Here's how the part is built. I have some questions about the finished solid (model axes, mm). A direction names the side the tool comes from. Give positions to 0.01 mm unless a question says otherwise; leave off trailing zeros. Order: outer loops, then holes, each group sorted by start corner. A loop starts at its lowest first (then second) coordinate and runs counter-clockwise, first axis right, second up. Notation, with made-up numbers: (8, 78.25) - (41, 78.25) arc R34 ccw to (41, 116.25) - close; hole circle Ø2 at (-27, -6.75). An arc over 180 degrees is marked (long way). One line per question, with ' | ' between items.
from build123d import *

# Parameters (mm, degrees)
SKETCH1_R           = 2
BOSS_EXTRUDE1_DEPTH = 3.3
SKETCH2_R           = 2
CUT_EXTRUDE1_DEPTH  = 513.420535354
SKETCH3_R           = 2
CUT_EXTRUDE2_DEPTH  = 4


with BuildPart() as part:
    # Sketch1 → Boss-Extrude1 (new body)
    with BuildSketch(Plane.XY):
        Polygon((327.436217585, 0.003466677), (121.498383462, 0.003466677), (108.169003487, 28.58841428), (-63.446663307, -51.437285405), (-52.881206764, -74.094980081), (-74.632593653, -84.237818363), (36.177914576, -321.871720124), (57.929301464, -311.728881842), (398.70102939, -152.824415428), align=None)
        with Locations(Location((372.759364157, -134.57831982, 0), (0, 0, 180))):
            Circle(SKETCH1_R, mode=Mode.SUBTRACT)
    extrude(amount=BOSS_EXTRUDE1_DEPTH)

    # Sketch2 → Cut-Extrude1 (cut, through all)
    with BuildSketch(Plane.XY.offset(3.3)):
        with Locations((105.144723808, 16.144390316)):
            Circle(SKETCH2_R)
        with Locations((-26.593400357, -45.286105853)):
            Circle(SKETCH2_R)
    extrude(amount=-CUT_EXTRUDE1_DEPTH, mode=Mode.SUBTRACT)

    # Sketch3 → Cut-Extrude2 (cut)
    with BuildSketch(Plane.XY.offset(3.3)):
        with Locations((45.851705082, -295.293199148)):
            Circle(SKETCH3_R)
        with Locations((63.977860822, -286.840833914)):
            Circle(SKETCH3_R)
    extrude(amount=-CUT_EXTRUDE2_DEPTH, mode=Mode.SUBTRACT)


solid = part.part
1) I'm going to push flat-ended pins straight in: P1, Ø1, axis at x = -18.5, y = -41, coming from the -Z side; P2, Ø3.5, axis at x = 63.98, y = -286.84, coming from the +Z side; P3, Ø1.5, axis at x = 280.5, z = 3, coming from the +Y side; P4, Ø1, axis at y = -181.5, z = 1, coming from the +X side. Where does each tip first touch, or does it pass through?
Model answer:
P1: stops at z = 0 | P2: passes through | P3: stops at y = 0 | P4: stops at x = 338.28
2) On a 3-axis mill with a long thin cutter (end or side, diameter ignored), from which of +Z, -Z, +X, -X, +Y, -Y can I reach the whole of each face in a straight line? I mean faces 1 (the face through (-20, -201.4, 1.6)), 2 (the face through (-63.605, -79.095, 1.627)). Say none if no direction works.
Model answer:
face 1: +Z, -Z, -X, -Y | face 2: +Z, -Z, -X
3) I want a section at C-C (x = 241). List the corners of the cut face in (y, z) for me.
Model answer:
outline: (-226.36, 0) - (0, 0) - (0, 3.3) - (-226.36, 3.3) - close
4) Please list where these lines run through material, in increasing order: L1, parallel to Y at x = 45, z = 2.85; L2, parallel to Y at x = 171, z = 1.1; L3, parallel to X at y = -31.5, z = 0.4.
Model answer:
L1: y = -317.76 to -297.1, -293.48 to -0.87 | L2: y = -259 to 0 | L3: x = -20.69 to 342.13
5) I want a section at B-B (y = -18.5). List the corners of the cut face in (x, z) for me.
Model answer:
outline: (7.19, 0) - (336.06, 0) - (336.06, 3.3) - (7.19, 3.3) - close
6) Thinking about a two-plate mould opening in Y: for faces 3 (the face through (-58.238, -62.608, 1.627)), 4 (the face through (363.567, -77.48, 1.627)), 5 (the face through (159, -144, 0)), which applies, +Y half, -Y half, draft (parallel to the pull), parting line (faces both ways), or undercut?
Model answer:
face 3: undercut | face 4: +Y half | face 5: draft
7) I want a section at A-A (z = 2.35). List the corners of the cut face in (x, y) for me.
Model answer:
outline: (-74.63, -84.24) - (36.18, -321.87) - (398.7, -152.82) - (327.44, 0) - (121.5, 0) - (108.17, 28.59) - (-63.45, -51.44) - (-52.88, -74.09) - close; hole circle Ø4 at (-26.59, -45.29); hole circle Ø4 at (45.85, -295.29); hole circle Ø4 at (63.98, -286.84); hole circle Ø4 at (105.14, 16.14); hole circle Ø4 at (372.76, -134.58)
